Answer from the drawing. Dimensions are ordinates in mm from the lowest x, y and z of the part. A direction names the side the tool comes from. Round coordinates to 2 decimals unless told otherwise and drop trailing zeros. Order: outer loops, then holes, each group sorted by start corner. A loop starts at its lowest first (then second) coordinate and runs counter-clockwise, first axis right, second up. Notation, with made-up numbers: M 17.5,33.5 L 61.5,33.5 A28 cw 61.5,59.5 Z; hole C 65,53.5 d9. An arc over 180 degrees is marked long. Answer as a JSON object with one key per item and string values. Group by question number.
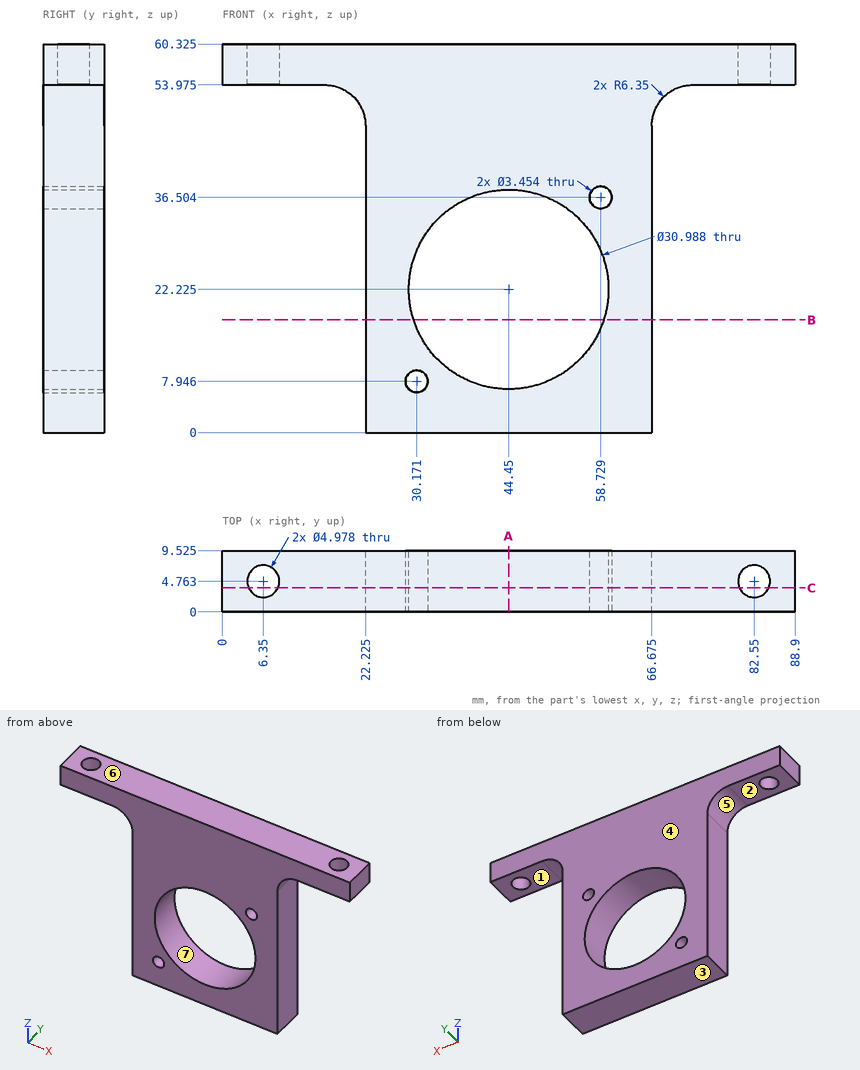
Item 1: Each of these flat-tipped pins is pushed along its axis until it touches: pin 1 (2 mm diameter, centred on y = 4.5, z = 22, fed in from -X) (1 decimal); pin 2 (3 mm diameter, centred on x = 82.5, y = 3.5, fed in from -Z) (1 decimal). Where does it stop, or does it pass through?
Item 2: A tool of negligible diameter and unlimited length cuts with its end or side. For the marked faces 1, 2 and 3, from which of +Z, -Z, +X, -X, +Y, -Y can it reach the whole face along a straight path? Write none if from no direction.
Item 3: Consider L1, parallel to Y at x = 6.35, z = 58 (1 decimal); L2, parallel to Z at x = 74, y = 0.5 (1 decimal); L3, parallel to X at y = 5.25, z = 5.5 (1 decimal). Determine where each line is inside the solid, lowest interval first.
Item 4: The mould has two halves that part along Z. Classify the marked faces 4, 5, 6 and 7: +Z half, -Z half, draft (parallel to the pull), parting line (faces both ways), or undercut.
Item 5: Find section C-C (y = 3.75). Give the number of separate pieces and of enclosed holes in the cut face, and give its area (3 significant figures).
Item 6: Find section A-A (x = 44.45). Give the vertices of the cut face in (y, z) (1 decimal).
Item 7: Find section B-B (z = 17.5). Give the vertices of the cut face in (x, y) (1 decimal).
Responses:
{
 "1": {"pin 1": "stops at x = 22.2", "pin 2": "stops at z = 54"},
 "2": {"face 1": "-Z, +X, +Y, -Y", "face 2": "-Z, -X, +Y, -Y", "face 3": "-Z, +X, -X, +Y, -Y"},
 "3": {"L1": "y = 0 to 2.3, 7.3 to 9.5", "L2": "z = 54 to 60.3", "L3": "x = 22.2 to 66.7"},
 "4": {"face 4": "draft", "face 5": "-Z half", "face 6": "+Z half", "face 7": "undercut"},
 "5": {"separate pieces": "3", "enclosed holes": "3", "area": "2,150 mm^2"},
 "6": {"outline": "M 0,0 L 9.5,0 L 9.5,6.7 L 0,6.7 Z; M 0,37.7 L 9.5,37.7 L 9.5,60.3 L 0,60.3 Z"},
 "7": {"outline": "M 22.2,0 L 29.7,0 L 29.7,9.5 L 22.2,9.5 Z; M 59.2,0 L 66.7,0 L 66.7,9.5 L 59.2,9.5 Z"}
}
